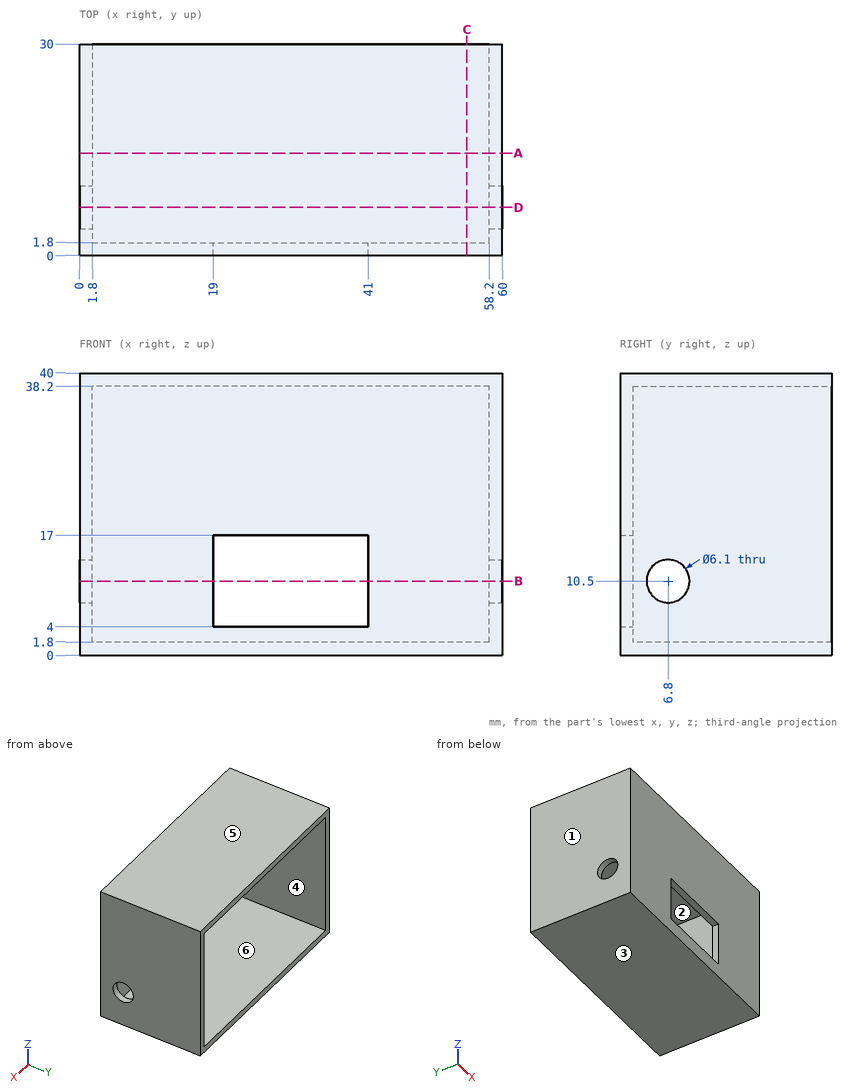
Print and shaded views of the part. All mm, measured from the part's lowest x, y and z. A direction names the side the tool comes from. Coordinates: 2 decimals unless noted, no trailing zeros. Loops run counter-clockwise (first coordinate to the right, second up) from the corner with the lowest first, then second, coordinate; pieces in that order, holes last. Notation, with made-up numbers: (-34.5, 73.25) - (-11.5, 73.25) arc R31 cw to (-11.5, 105.25) - close; hole circle Ø2 at (7.5, 15). An arc over 180 degrees is marked (long way). Write item = value, one per line. Start each with the question number.
Item 1: Cut at D-D, the plane y = 6.8. Give the cut face in (x, z), and give its area (3 significant figures).
Item 2: Mould opens along X. For the marked faces 1, 2, 3 and 4 say: released by +X, released by -X, zero draft, split by the parting line, or undercut.
Item 3: Cut at A-A, the plane y = 14.5. Give the cut face in (x, z), and give its area (3 significant figures).
Item 4: Flat gauge pin, fed straight in: pin 1 Ø1.5 at (x, z) = (46.5, 14) entering from +Y. Where does the tip first touch, or does it go through?
Item 5: 3-axis set-ups, long thin cutter, end or side, ignore diameter. For the marked faces 5 and 6: which of +Z, -Z, +X, -X, +Y, -Y reach the whole face in a straight line?
Item 6: Cut at B-B, the plane z = 10.5. Give the cut face in (x, y), and give its area (3 significant figures).
Item 7: Cut at C-C, the plane x = 55. Give the cut face in (y, z), and give its area (3 significant figures).
Item 8: Wall check: L1, parallel to Y at x = 59.2, z = 10.5; L2, parallel to X at y = 9.75, z = 16; L3, parallel to Z at x = 39, y = 20.25. Give the ranges that are in metal, low to high. Write a range as from..to.
The answers:
q1.outline = (0, 0) - (60, 0) - (60, 7.45) - (58.2, 7.45) - (58.2, 1.8) - (1.8, 1.8) - (1.8, 7.45) - (0, 7.45) - close; (0, 13.55) - (1.8, 13.55) - (1.8, 38.2) - (58.2, 38.2) - (58.2, 13.55) - (60, 13.55) - (60, 40) - (0, 40) - close
q1.area = 325 mm2
q2.face_1 = released by -X
q2.face_2 = undercut
q2.face_3 = zero draft
q2.face_4 = undercut
q3.outline = (0, 0) - (60, 0) - (60, 40) - (0, 40) - close; hole (1.8, 1.8) - (58.2, 1.8) - (58.2, 38.2) - (1.8, 38.2) - close
q3.area = 347 mm2
q4.pin_1 = 1.8
q5.face_5 = +Z, +X, -X, +Y, -Y
q5.face_6 = +Y
q6.outline = (0, 0) - (19, 0) - (19, 1.8) - (1.8, 1.8) - (1.8, 3.75) - (0, 3.75) - close; (0, 9.85) - (1.8, 9.85) - (1.8, 30) - (0, 30) - close; (41, 0) - (60, 0) - (60, 3.75) - (58.2, 3.75) - (58.2, 1.8) - (41, 1.8) - close; (58.2, 9.85) - (60, 9.85) - (60, 30) - (58.2, 30) - close
q6.area = 148 mm2
q7.outline = (0, 0) - (30, 0) - (30, 1.8) - (1.8, 1.8) - (1.8, 38.2) - (30, 38.2) - (30, 40) - (0, 40) - close
q7.area = 174 mm2
q8.L1 = 0..3.75, 9.85..30
q8.L2 = 0..1.8, 58.2..60
q8.L3 = 0..1.8, 38.2..40
